from build123d import *

# Parameters (mm, degrees)
ESQUISSE1_W                                   = 30
ESQUISSE1_H                                   = 26
ESQUISSE1_R                                   = 11
BOSS_EXTRU_1_DEPTH                            = 5
TROU_POUR_TARAUDAGE_POUR_TROU_TARAUD_M2_D     = 1.6
TROU_POUR_TARAUDAGE_POUR_TROU_TARAUD_M2_DEPTH = 5
TROU_POUR_TARAUDAGE_POUR_TROU_TARAUD_M2_TIP   = 0.480688495
TROU_POUR_TARAUDAGE_POUR_TROU_TARAUD_2_D      = 1.6
TROU_POUR_TARAUDAGE_POUR_TROU_TARAUD_2_DEPTH  = 5
TROU_POUR_TARAUDAGE_POUR_TROU_TARAUD_2_TIP    = 0.480688495


with BuildPart() as part:
    # Esquisse1 → Boss.-Extru.1 (new body)
    with BuildSketch(Plane.XY):
        with Locations((15, 13)):
            Rectangle(ESQUISSE1_W, ESQUISSE1_H)
        with Locations((15, 13)):
            Circle(ESQUISSE1_R, mode=Mode.SUBTRACT)
    extrude(amount=BOSS_EXTRU_1_DEPTH)

    # Trou pour taraudage pour trou taraud_ M2
    with Locations(Plane(origin=(0, 26, 0), x_dir=(1, 0, 0), z_dir=(0, 1, 0))):
        with Locations((4, -2.5), (26, -2.5)):
            Hole(TROU_POUR_TARAUDAGE_POUR_TROU_TARAUD_M2_D / 2, depth=TROU_POUR_TARAUDAGE_POUR_TROU_TARAUD_M2_DEPTH)
            with Locations((0, 0, -(TROU_POUR_TARAUDAGE_POUR_TROU_TARAUD_M2_DEPTH + TROU_POUR_TARAUDAGE_POUR_TROU_TARAUD_M2_TIP / 2))):  # 118° drill point
                Cone(0, TROU_POUR_TARAUDAGE_POUR_TROU_TARAUD_M2_D / 2, TROU_POUR_TARAUDAGE_POUR_TROU_TARAUD_M2_TIP, mode=Mode.SUBTRACT)

    # Trou pour taraudage pour trou taraud 2
    with Locations(Plane(origin=(0, 0, 0), x_dir=(-1, 0, 0), z_dir=(0, -1, 0))):
        with Locations((-4, -2.5), (-26, -2.5)):
            Hole(TROU_POUR_TARAUDAGE_POUR_TROU_TARAUD_2_D / 2, depth=TROU_POUR_TARAUDAGE_POUR_TROU_TARAUD_2_DEPTH)
            with Locations((0, 0, -(TROU_POUR_TARAUDAGE_POUR_TROU_TARAUD_2_DEPTH + TROU_POUR_TARAUDAGE_POUR_TROU_TARAUD_2_TIP / 2))):  # 118° drill point
                Cone(0, TROU_POUR_TARAUDAGE_POUR_TROU_TARAUD_2_D / 2, TROU_POUR_TARAUDAGE_POUR_TROU_TARAUD_2_TIP, mode=Mode.SUBTRACT)


solid = part.part
Design review of the part built by this model. Coordinates are the model's own, in mm. A direction names the side the tool comes from. Coordinates: 2 decimals unless noted, no trailing zeros. Write each loop counter-clockwise with the first axis right and the second up, starting at its lowest first coordinate (ties: lowest second). Pieces come first, ordered by that corner, then holes. Notation, with made-up numbers: (-12.75, -39) - (38.25, -39) arc R20 ccw to (38.25, -2) - close; hole circle Ø11 at (31.25, 28.25). An arc over 180 degrees is marked (long way). Use one line per item in the form item = value.
Q1. Machinability: for faces 5 (the cylindrical face through (12.62, 2.26, 2.46)), 6 (the cylindrical face through (26.763, 2.535, 2.26)), 7 (the cylindrical face through (4.8, 23.5, 2.5)), which of the approach directions +Z, -Z, +X, -X, +Y, -Y give a long, thin tool a straight path to every point of the face, cutting with its end or side? Answer none if there is none.
Taken from the geometry:
face_5 = +Z, -Z
face_6 = -Y
face_7 = +Y
Q2. For probe 1 along X at (y, z) = (24.9, 2.5); probe 2 along Y at (x, z) = (15, 3.9); probe 3 along Z at (x, y) = (4, 24.8), list the stretches that pass through material, from the lowest coordinate up.
Taken from the geometry:
probe_1 = 0 to 3.2, 4.8 to 25.2, 26.8 to 30
probe_2 = 0 to 2, 24 to 26
probe_3 = 0 to 1.7, 3.3 to 5
Q3. Consider section B-B (y = 13). Write out the cut boundary in (x, z), plus the area to 3 significant figures.
Taken from the geometry:
outline = (0, 0) - (4, 0) - (4, 5) - (0, 5) - close; (26, 0) - (30, 0) - (30, 5) - (26, 5) - close
area = 40.0 mm^2
Q4. Consider section A-A (x = 15). Write out the cut boundary in (y, z), plus the area to 3 significant figures.
Taken from the geometry:
outline = (0, 0) - (2, 0) - (2, 5) - (0, 5) - close; (24, 0) - (26, 0) - (26, 5) - (24, 5) - close
area = 20.0 mm^2
Q5. Insertion check: pin 1 Ø2.5 at (x, z) = (4, 2.5) entering from -Y; pin 2 Ø1.4 at (x, z) = (4, 2.5) entering from -Y; pin 3 Ø1 at (x, z) = (26, 2.5) entering from -Y. Each pin has a flat end and moves straight along its axis. Give the tip position at first contact, or say it passes through.
Taken from the geometry:
pin_1 = 0
pin_2 = 5.06
pin_3 = 5.18
Q6. The part is to be moulded in two halves that separate along X. For faces 1 (the flat face through (15, 0, 2)), 2 (the flat face through (30, 13, 2)), 3 (the conical face through (3.94, 5.4, 2.62)), 4 (the flat face through (0, 13, 2)), say which applies: +X half, -X half, draft (parallel to the pull), parting line (faces both ways), or undercut.
Taken from the geometry:
face_1 = draft
face_2 = +X half
face_3 = undercut
face_4 = -X half
